Part model, mm, in its own coordinate system. Face numbers are marked on the shaded views. A direction names the side the tool comes from. Give positions to 0.01 mm unless a question says otherwise; leave off trailing zeros. Order: outer loops, then holes, each group sorted by start corner. A loop starts at its lowest first (then second) coordinate and runs counter-clockwise, first axis right, second up. Notation, with made-up numbers: M 67.5,79 L 72.5,79 A15 cw 72.5,101 Z; hole C 29,23 d2. An arc over 180 degrees is marked long. One line per question, with ' | ' between items.
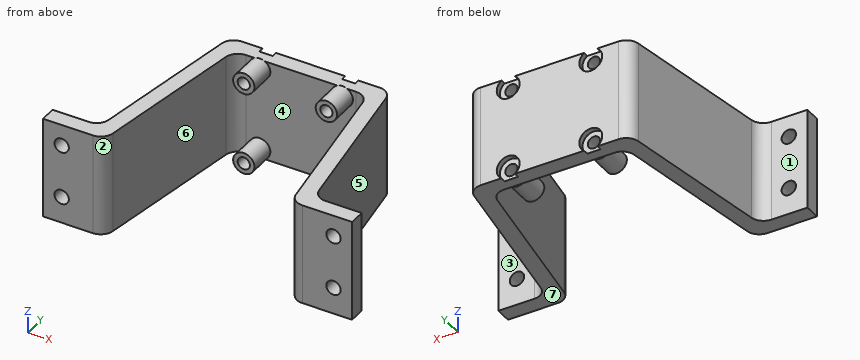
```python
from build123d import *

# Parameters (mm, degrees)
EXTRUDE_1_DEPTH     = 9.5
SKETCH_2_R          = 1.15
CUT_EXTRUDE_1_DEPTH = 45.58138625
EXTRUDE_START       = 5
SKETCH_3_R          = 2
SKETCH_3_R_2        = 1.15
EXTRUDE_2_DEPTH     = 5
SKETCH_4_R          = 1.35
CUT_EXTRUDE_2_DEPTH = 45.634672722
FILLET_1_R          = 2.5
SKETCH_5_R          = 2.15
CUT_EXTRUDE_3_DEPTH = 1


with BuildPart() as part:
    # 草图1 → 凸台-拉伸1 (new, symmetric)
    with BuildSketch(Plane.XY):
        Polygon((-20.07375687, 0), (-15.07375687, 32.5), (15.07375687, 32.5), (20.07375687, 0), (29, 0), (29, -3), (17.5, -3), (12.5, 29.5), (-12.5, 29.5), (-17.5, -3), (-29, -3), (-29, 0), align=None)
    extrude(amount=EXTRUDE_1_DEPTH, both=True)

    # 草图2 → 切除-拉伸1 (cut, through all)
    with BuildSketch(Plane.XZ.offset(-29.5)):
        with Locations(Location((-7.747, 7.747, 0), (0, 0, 270))):
            Circle(SKETCH_2_R)
        with Locations(Location((7.747, 7.747, 0), (0, 0, 270))):
            Circle(SKETCH_2_R)
        with Locations(Location((7.747, -7.747, 0), (0, 0, 270))):
            Circle(SKETCH_2_R)
        with Locations(Location((-7.747, -7.747, 0), (0, 0, 270))):
            Circle(SKETCH_2_R)
    extrude(amount=-CUT_EXTRUDE_1_DEPTH, mode=Mode.SUBTRACT)

    # 草图3 → 凸台-拉伸2 (add)
    # profile 1 of 4: a face of its own
    with BuildSketch(Plane.XZ.offset(-29.5).offset(EXTRUDE_START)):
        with Locations(Location((-7.747, 7.747, 0), (0, 0, 118.776999733))):
            Circle(SKETCH_3_R)
        with Locations(Location((-7.747, 7.747, 0), (0, 0, 270))):
            Circle(SKETCH_3_R_2, mode=Mode.SUBTRACT)
    # profile 2 of 4: a face of its own
    with BuildSketch(Plane.XZ.offset(-29.5).offset(EXTRUDE_START)):
        with Locations(Location((7.747, 7.747, 0), (0, 0, 118.776999733))):
            Circle(SKETCH_3_R)
        with Locations(Location((7.747, 7.747, 0), (0, 0, 270))):
            Circle(SKETCH_3_R_2, mode=Mode.SUBTRACT)
    # profile 3 of 4: a face of its own
    with BuildSketch(Plane.XZ.offset(-29.5).offset(EXTRUDE_START)):
        with Locations(Location((7.747, -7.747, 0), (0, 0, 241.223000267))):
            Circle(SKETCH_3_R)
        with Locations(Location((7.747, -7.747, 0), (0, 0, 270))):
            Circle(SKETCH_3_R_2, mode=Mode.SUBTRACT)
    # profile 4 of 4: a face of its own
    with BuildSketch(Plane.XZ.offset(-29.5).offset(EXTRUDE_START)):
        with Locations(Location((-7.747, -7.747, 0), (0, 0, 241.223000267))):
            Circle(SKETCH_3_R)
        with Locations(Location((-7.747, -7.747, 0), (0, 0, 270))):
            Circle(SKETCH_3_R_2, mode=Mode.SUBTRACT)
    extrude(amount=-EXTRUDE_2_DEPTH)

    # 草图4 → 切除-拉伸2 (cut, through all)
    with BuildSketch(Plane(origin=(0, 0, 0), x_dir=(1, 0, 0), z_dir=(0, 1, 0))):
        with Locations(Location((-25.5, 4.5, 0), (0, 0, 180))):
            Circle(SKETCH_4_R)
        with Locations(Location((-25.5, -5.5, 0), (0, 0, 180))):
            Circle(SKETCH_4_R)
        with Locations(Location((25.5, 4.5, 0), (0, 0, 180))):
            Circle(SKETCH_4_R)
        with Locations(Location((25.5, -5.5, 0), (0, 0, 180))):
            Circle(SKETCH_4_R)
    extrude(amount=-CUT_EXTRUDE_2_DEPTH, mode=Mode.SUBTRACT)

    # 圆角1
    fillet_1_edges = [part.edges().sort_by_distance(p)[0] for p in [
        (-20.07375687, 0, 0),
        (-15.07375687, 32.5, 0),
        (15.07375687, 32.5, 0),
        (20.07375687, 0, 0),
        (17.5, -3, 0),
        (12.5, 29.5, 0),
        (-12.5, 29.5, 0),
        (-17.5, -3, 0),
    ]]
    fillet(fillet_1_edges, radius=FILLET_1_R)

    # 草图5 → 切除-拉伸3 (cut)
    with BuildSketch(Plane(origin=(0, 32.5, 0), x_dir=(1, 0, 0), z_dir=(0, 1, 0))):
        with Locations((-7.747, -7.747)):
            Circle(SKETCH_5_R)
        with Locations((7.747, -7.747)):
            Circle(SKETCH_5_R)
        with Locations((7.747, 7.747)):
            Circle(SKETCH_5_R)
        with Locations((-7.747, 7.747)):
            Circle(SKETCH_5_R)
    extrude(amount=-CUT_EXTRUDE_3_DEPTH, mode=Mode.SUBTRACT)


solid = part.part
```
1. Drop flat-ended pins along their axis: pin 1 (1.6 mm diameter, centred on x = 25.5, z = -4.5, fed in from -Y); pin 2 (3.5 mm diameter, centred on x = -7.747, z = 7.747, fed in from +Y); pin 3 (3 mm diameter, centred on x = 7.747, z = 7.747, fed in from -Y); pin 4 (3 mm diameter, centred on x = -16, y = 22.5, fed in from -Z). Give the stop position or say it passes through.
Worked out:
pin 1: passes through | pin 2: stops at y = 31.5 | pin 3: stops at y = 24.5 | pin 4: stops at z = -9.5
2. Mould opens along X. For the marked faces 5, 6 and 7 say: released by +X, released by -X, zero draft, split by the parting line, or undercut.
Worked out:
face 5: released by +X | face 6: undercut | face 7: zero draft
3. Slice it at B-B on z = -4.5. Give the cut face in (x, y), then the cut area to 3 significant figures.
Worked out:
outline: M -29,-3 L -26.85,-3 L -26.85,0 L -29,0 Z; M -24.15,-3 L -19.64,-3 A2.5 ccw -17.17,-0.88 L -12.83,27.38 A2.5 cw -10.36,29.5 L 10.36,29.5 A2.5 cw 12.83,27.38 L 17.17,-0.88 A2.5 ccw 19.64,-3 L 24.15,-3 L 24.15,0 L 22.22,0 A2.5 cw 19.75,2.12 L 15.4,30.38 A2.5 ccw 12.93,32.5 L -12.93,32.5 A2.5 ccw -15.4,30.38 L -19.75,2.12 A2.5 cw -22.22,0 L -24.15,0 Z; M 26.85,-3 L 29,-3 L 29,0 L 26.85,0 Z | area: 325 mm2
4. Tool access for the marked faces 1, 2, 3 and 4: list every direction of +Z, -Z, +X, -X, +Y, -Y with a clear straight run to the whole face (end or side of a thin tool).
Worked out:
face 1: +Z, -Z, -X, +Y | face 2: +Z, -Z, -Y | face 3: +Z, -Z, +X, +Y | face 4: -Y
5. Slice it at C-C on y = 20. Give the cut face in (x, z).
Worked out:
outline: M -17,-9.5 L -13.96,-9.5 L -13.96,9.5 L -17,9.5 Z; M 13.96,-9.5 L 17,-9.5 L 17,9.5 L 13.96,9.5 Z
6. Slice it at A-A on x = -25.5. Give the cut face in (y, z), then the cut area to 3 significant figures.
Worked out:
outline: M -3,-9.5 L 0,-9.5 L 0,-5.85 L -3,-5.85 Z; M -3,-3.15 L 0,-3.15 L 0,4.15 L -3,4.15 Z; M -3,6.85 L 0,6.85 L 0,9.5 L -3,9.5 Z | area: 40.8 mm2
7. Slice it at D-D on y = 1.5. Give the cut face in (x, z).
Worked out:
outline: M -19.93,-9.5 L -16.81,-9.5 L -16.81,9.5 L -19.93,9.5 Z; M 16.81,-9.5 L 19.93,-9.5 L 19.93,9.5 L 16.81,9.5 Z
8. Probe L1, parallel to Z at x = -25, y = -1; L2, parallel to X at y = 27, z = 7.5; L3, parallel to X at y = 21, z = -4. List the from-to ranges inside material, lowest first. Write a range as from..to.
Worked out:
L1: z = -9.5..-5.75, -3.25..4.25, 6.75..9.5 | L2: x = -15.92..-12.88, -9.73..-8.87, -6.62..-5.76, 5.76..6.62, 8.87..9.73, 12.88..15.92 | L3: x = -16.84..-13.81, 13.81..16.84
